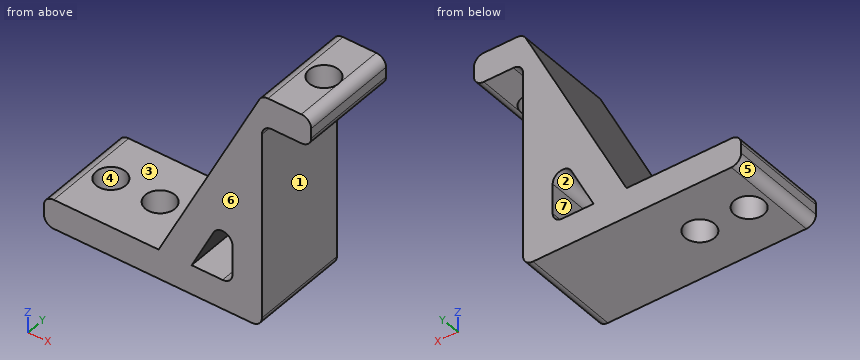
Autodesk Inventor part; units mm, degrees
ref_plane "YZ Plane" through (0, 0, 0) normal (1, 0, 0) x (0, 1, 0)
ref_plane "XZ Plane" through (0, 0, 0) normal (0, 1, 0) x (-1, 0, 0)
ref_plane "XY Plane" through (0, 0, 0) normal (0, 0, 1) x (1, 0, 0)
sketch "Sketch1" plane through (0, 0, 0) normal (0, 1, 0) x (-1, 0, 0)
  line L0 (0, 0) -> (0, -48)
  line L1 (0, -48) -> (24, -48)
  line L2 (24, -48) -> (0, 0)
  line L3 (6, -25.4164) -> (6, -42)
  line L4 (6, -42) -> (14.2918, -42)
  line L5 (14.2918, -42) -> (6, -25.4164)
  line L6 (0, 0) -> (-10, 0)
  line L7 (-10, 0) -> (-10, -6)
  line L8 (-10, -6) -> (0, -6)
  line L9 (0, -6) -> (0, 0)
  dimension "d0" = 48
  dimension "d1" = 24
  dimension "d4" = 6
  dimension "d5" = 10
  dimension "d6" = 6
extrude "Extrusion1" add sketch "Sketch1" along normal blind 20
sketch "Sketch2" plane through (0, 0, 0) normal (0, 0, 1) x (1, 0, 0)
  circle A0 centre (5, 10) radius 3
  line L0 (0, 0) -> (10, 0)
  line L1 (0, 0) -> (0, 20)
  dimension "d9" = 6
  dimension "d10" = 10
  dimension "d11" = 5
extrude "Extrusion2" cut sketch "Sketch2" against normal through all
sketch "Sketch3" plane through (0, 0, 0) normal (0, -1, 0) x (1, 0, 0)
  line L0 (-14.2918, -42) -> (-6, -42)
  line L1 (-14.2918, -42) -> (-44.2918, -42)
  line L2 (-44.2918, -42) -> (-19.2918, -42)
  line L3 (-19.2918, -42) -> (-19.2918, -48)
  line L4 (-19.2918, -48) -> (-44.2918, -48)
  line L5 (-44.2918, -48) -> (-44.2918, -42)
  point P0 (0, 0)
  dimension "d14" = 30
  dimension "d15" = 25
  dimension "d16" = 6
extrude "Extrusion3" add sketch "Sketch3" against normal blind 20
sketch "Sketch4" plane through (0, 0, -48) normal (0, 0, -1) x (-1, 0, 0)
  circle A0 centre (38.2918, 10) radius 3
  circle A1 centre (28.2918, 10) radius 3
  line L0 (44.2918, 0) -> (44.2918, 20)
  line L1 (0, 0) -> (44.2918, 0)
  dimension "d19" = 6
  dimension "d20" = 6
  dimension "d21" = 6
  dimension "d22" = 10
  dimension "d23" = 10
  dimension "d24" = 10
extrude "Extrusion4" cut sketch "Sketch4" against normal through all
fillet "Fillet1" radius 2 2 edges at (-6, 10, -42) (-6, 10, -25.4164)
fillet "Fillet2" radius 2 3 edges at (0, 10, -48) (-44.2918, 10, -48) (-44.2918, 10, -42)
fillet "Fillet3" radius 2 1 edges at (0, 10, -6)
fillet "Fillet4" radius 2 3 edges at (10, 10, 0) (10, 10, -6) (0, 10, 0)
properties part number "RightAngle_PulleySupport"
Check sheet for the modelled part. Datum: model origin and axes. Units: mm. Face numbers are marked on the shaded views. A direction names the side the tool comes from. Round coordinates to 2 decimals unless told otherwise and drop trailing zeros. Write each loop counter-clockwise with the first axis right and the second up, starting at its lowest first coordinate (ties: lowest second). Pieces come first, ordered by that corner, then holes. Notation, with made-up numbers: M -29.5,86.5 L -4.5,86.5 A21 ccw -4.5,125.5 Z; hole C 42.25,80.25 d2. An arc over 180 degrees is marked long. Write item = value, one per line. Start each with the question number.
1. Section check A-A, the plane y = 10. State how many separate pieces and enclosed holes the cut face has, then the cut area to 3 significant figures.
2. Scan lines: line 1 (Y direction, x = 5, z = -4.1); line 2 (Z direction, x = -26, y = 3.5); line 3 (Z direction, x = 4.5, y = 6). Record each from-to range of solid material in increasing order. Write a range as [from, to].
3. Gauge pin test, flat ends, axial feed: pin 1 (1 mm diameter, centred on y = 9.5, z = -31.5, fed in from +X); pin 2 (4 mm diameter, centred on x = -14.5, y = 8.5, fed in from +Z); pin 3 (7 mm diameter, centred on x = -28.29, y = 10, fed in from +Z). Record the tip position at first contact, or that the pin passes through.
4. Tool access check on the marked faces 1, 2 and 3. Record the directions out of +Z, -Z, +X, -X, +Y, -Y that give a thin tool (end or side, any length) a straight path to the whole face; none if there is none.
5. Section check C-C, the plane y = 16.5. Record the cut outline in (x, z), then the cut area to 3 significant figures.
6. Section check D-D, the plane z = -37.5. Record the cut outline in (x, y).
7. Section check B-B, the plane x = 5. Record the cut outline in (y, z).
8. Release check for a two-part mould opening along X. For the marked faces 4, 5, 6 and 7 record: pulls with the +X half, pulls with the -X half, needs draft (parallel to the pull), parting line crosses it, or undercut.
Results found:
q1.separate_pieces = 4
q1.enclosed_holes = 1
q1.area = 599 mm^2
q2.line_1 = [0, 7], [13, 20]
q2.line_2 = [-48, -42]
q2.line_3 = [-6, 0]
q3.pin_1 = 0
q3.pin_2 = -25
q3.pin_3 = -42
q4.face_1 = -Z, +X, +Y, -Y
q4.face_2 = +Y, -Y
q4.face_3 = +Z, -X, +Y, -Y
q5.outline = M -44.29,-46 A2 ccw -42.29,-48 L -2,-48 A2 ccw 0,-46 L 0,-8 A2 cw 2,-6 L 8,-6 A2 ccw 10,-4 L 10,-2 A2 ccw 8,0 L 1.24,0 A2 ccw -0.55,-1.11 L -21,-42 L -42.29,-42 A2 ccw -44.29,-44 Z; hole M -14.29,-42 L -8,-42 A2 ccw -6,-40 L -6,-33.89 A2 ccw -9.79,-32.99 Z
q5.area = 707 mm^2
q6.outline = M -18.75,0 L -12.04,0 L -12.04,20 L -18.75,20 Z; M -6,0 L 0,0 L 0,20 L -6,20 Z
q7.outline = M 0,-6 L 7,-6 L 7,0 L 0,0 Z; M 13,-6 L 20,-6 L 20,0 L 13,0 Z
q8.face_4 = undercut
q8.face_5 = pulls with the -X half
q8.face_6 = needs draft
q8.face_7 = undercut
